For this review, take the finished solid that the model builds, in its own axes (mm). Face numbers are marked on the shaded views. A direction names the side the tool comes from. Round coordinates to 2 decimals unless told otherwise and drop trailing zeros. Write each loop counter-clockwise with the first axis right and the second up, starting at its lowest first coordinate (ties: lowest second). Pieces come first, ordered by that corner, then holes. Notation, with made-up numbers: (68, 47) -> (101, 47) arc R18 cw to (101, 63) -> close; hole circle Ø10 at (-11, 34). An arc over 180 degrees is marked (long way). Answer in a Markdown table with one row per item. Add a question column.
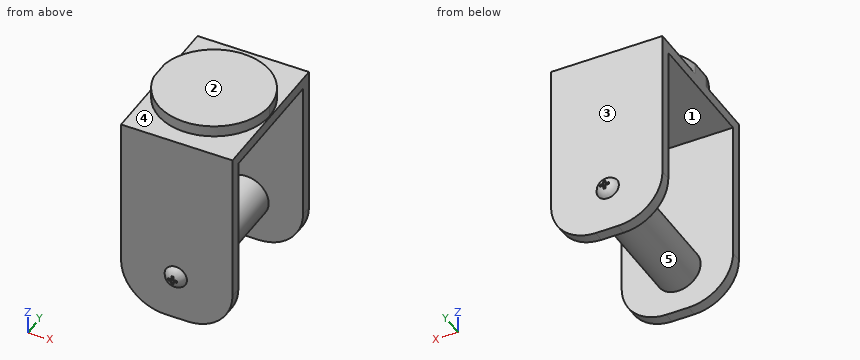
```python
from build123d import *

# Parameters (mm, degrees)
F1_DEPTH  = 5
F2_W      = 50
F2_H      = 55
F2_H_2    = 5
F3_DEPTH  = 5
F7_DEPTH  = 5
F8_R      = 10
F9_DEPTH  = 55
F10_R     = 5
F11_DEPTH = 3
F12_W     = 1.5
F12_H     = 1
F12_W_2   = 1
F12_H_2   = 1.5
F14_DEPTH = 3
F15_R     = 5
F16_DEPTH = 3
F18_DEPTH = 3


# Not quite as in the source:
# - a fillet or chamfer that OpenCascade refuses, or shapes differently, is made with other operations: its cross-section is extruded or revolved along the edge and cut away or added


with BuildPart() as f1:
    # F0 (on Front) → F1 (new body)
    with BuildSketch(Plane.XZ):
        with BuildLine():
            Line((25.4373252392, 36.0385786295), (-24.5626747608, 36.0385786295))
            Line((-24.5626747608, 36.0385786295), (-24.5626747608, -26.9614213705))
            ThreePointArc((-24.5626747608, -26.9614213705), (-18.7048103845, -41.1035569942), (-4.5626747608, -46.9614213705))
            Line((-4.5626747608, -46.9614213705), (5.4373252392, -46.9614213705))
            ThreePointArc((5.4373252392, -46.9614213705), (19.5794608629, -41.1035569942), (25.4373252392, -26.9614213705))
            Line((25.4373252392, -26.9614213705), (25.4373252392, 36.0385786295))
        make_face()
    extrude(amount=F1_DEPTH)

    # F2 (on face) → F3 (join)
    with BuildSketch(Plane.XY.offset(36.0385786295)):
        with Locations((0.4373252392, 27.5)):
            Rectangle(F2_W, F2_H)
        with Locations((0.4373252392, -2.5)):
            Rectangle(F2_W, F2_H_2)
    extrude(amount=F3_DEPTH)

    # F5: F1 across plane


with BuildPart() as f1_1:
    add(f1.part)
    add(f1.part.mirror(Plane(origin=(0.4373252392, 27.5, -3.8633044256), x_dir=(1, 0, 0), z_dir=(0, 1, 0))))

    # F6 (on face) → F7 (join)
    with BuildSketch(Plane.XY.offset(41.0385786295)):
        with BuildLine():
            ThreePointArc((-24.5626747608, 22.8443573382), (2.3380687521, 2.6095714278), (25, 27.5))
            ThreePointArc((25, 27.5), (2.3380687521, 52.3904285722), (-24.5626747608, 32.1556426618))
            Line((-24.5626747608, 32.1556426618), (-24.5626747608, 22.8443573382))
        make_face()
    extrude(amount=F7_DEPTH)

    # F8 (on face) → F9 (join, through all)
    with BuildSketch(Plane(origin=(0, 0, 0), x_dir=(-1, 0, 0), z_dir=(0, 1, 0))):
        with Locations((0, -26.9662032763)):
            Circle(F8_R)
    extrude(amount=F9_DEPTH)

    # F10 (on face) → F11 (join)
    with BuildSketch(Plane.XZ.offset(5)):
        with Locations((0, -26.4660866176)):
            Circle(F10_R)
    extrude(amount=F11_DEPTH)

    # F13: fillet of radius 5 on 1 edges, made by hand

    # F13_s1 → F13_t2 (revolve, cut)
    with BuildSketch(Plane.XY.offset(-26.4660866176)):
        with BuildLine():
            ThreePointArc((5, -5), (3.1560370926, -7.1833001327), (0.417424305, -8))
            Line((0.417424305, -8), (5, -8))
            Line((5, -8), (5, -5))
        make_face()
    revolve(axis=Axis((0, -8, -26.4660866176), (0, -1, 0)), mode=Mode.SUBTRACT)

    # F12 (on face) → F14 (cut)
    with BuildSketch(Plane.XZ.offset(8)):
        with Locations((-1.25, -26.4660866176)):
            Rectangle(F12_W, F12_H)
        Polygon((1, -25.9660866176), (0.5, -25.9660866176), (0.5, -26.9660866176), (1, -26.9660866176), (2, -26.9660866176), (2, -25.9660866176), align=None)
        with Locations((0, -26.4660866176)):
            Rectangle(F12_W_2, F12_H)
        with Locations((0, -25.2160866176)):
            Rectangle(F12_W_2, F12_H_2)
        with Locations((0, -27.7160866176)):
            Rectangle(F12_W_2, F12_H_2)
    extrude(amount=-F14_DEPTH, mode=Mode.SUBTRACT)

    # F15 (on face) → F16 (join)
    with BuildSketch(Plane(origin=(0, 60, 0), x_dir=(-1, 0, 0), z_dir=(0, 1, 0))):
        with Locations((0, -26.4660866176)):
            Circle(F15_R)
    extrude(amount=F16_DEPTH)

    # F17 (on face) → F18 (cut)
    with BuildSketch(Plane(origin=(0, 63, 0), x_dir=(-1, 0, 0), z_dir=(0, 1, 0))):
        Polygon((0.5, -24.4660866176), (-0.5, -24.4660866176), (-0.5, -25.9660866176), (-2, -25.9660866176), (-2, -26.9660866176), (-0.5, -26.9660866176), (-0.5, -28.4660866176), (0.5, -28.4660866176), (0.5, -26.9660866176), (2, -26.9660866176), (2, -25.9660866176), (0.5, -25.9660866176), align=None)
    extrude(amount=-F18_DEPTH, mode=Mode.SUBTRACT)

    # F19: fillet of radius 5 on 1 edges, made by hand

    # F19_s1 → F19_t2 (revolve, cut)
    with BuildSketch(Plane.XY.offset(-26.4660866176)):
        with BuildLine():
            ThreePointArc((-5, 60), (-3.1560370926, 62.1833001327), (-0.417424305, 63))
            Line((-0.417424305, 63), (-5, 63))
            Line((-5, 63), (-5, 60))
        make_face()
    revolve(axis=Axis((0, 63, -26.4660866176), (0, 1, 0)), mode=Mode.SUBTRACT)


solid = f1_1.part
```
1. We need section D-D (y = 29.5). Write out the cut boundary in (x, z), plus the area to 3 significant figures.
2. For L1, parallel to Y at x = -6, z = -9; L2, parallel to Z at x = -0.5, y = 45.5; L3, parallel to Z at x = 23.5, y = 29, list the stretches that pass through material, from the lowest coordinate up. Write a range as [from, to].
3. The part is to be moulded in two halves that separate along Y. For the marked faces 1, 2 and 3, say which applies: pulls with the +Y half, pulls with the -Y half, needs draft (parallel to the pull), parting line crosses it, or undercut.
4. Clearance check with flat-ended pins moving along their axes: pin 1 Ø0.8 at (x, y) = (0, 62) entering from +Z; pin 2 Ø10 at (x, z) = (-13.5, 30.5) entering from -Y; pin 3 Ø6 at (x, z) = (7.5, -7) entering from +Y. State where each tip first meets the part, or that it passes through.
5. Tool access review of the marked faces 4 and 5: name each direction out of +Z, -Z, +X, -X, +Y, -Y from which nothing blocks a thin tool from reaching the whole face with its end or side.
6. We need section A-A (y = 50). Write out the cut boundary in (x, z).
7. We need section C-C (z = -35). Write out the cut boundary in (x, y).
8. We need section B-B (x = -8.5). Write out the cut boundary in (y, z), plus the area to 3 significant figures.
Response:
| question | item | result |
|---|---|---|
| 1 | outline | (-24.56, 36.04) -> (25.44, 36.04) -> (25.44, 41.04) -> (24.92, 41.04) -> (24.92, 46.04) -> (-24.56, 46.04) -> close; circle Ø20 at (0, -26.97) |
| 1 | area | 812 mm2 |
| 2 | L1 | [-5, 0], [55, 60] |
| 2 | L2 | [-36.95, -16.98], [36.04, 46.04] |
| 2 | L3 | [36.04, 46.04] |
| 3 | face 1 | undercut |
| 3 | face 2 | needs draft |
| 3 | face 3 | pulls with the +Y half |
| 4 | pin 1 | z = -22.58 |
| 4 | pin 2 | y = -5 |
| 4 | pin 3 | y = 60 |
| 5 | face 4 | +Z |
| 5 | face 5 | none |
| 6 | outline | (-24.56, 36.04) -> (25.44, 36.04) -> (25.44, 41.04) -> (10.9, 41.04) -> (10.9, 46.04) -> (-10.9, 46.04) -> (-10.9, 41.04) -> (-24.56, 41.04) -> close; circle Ø20 at (0, -26.97) |
| 7 | outline | (-22.88, -5) -> (23.75, -5) -> (23.75, 0) -> (5.95, 0) -> (5.95, 55) -> (23.75, 55) -> (23.75, 60) -> (-22.88, 60) -> (-22.88, 55) -> (-5.95, 55) -> (-5.95, 0) -> (-22.88, 0) -> close |
| 8 | outline | (-5, -46.57) -> (0, -46.57) -> (0, -32.23) -> (55, -32.23) -> (55, -46.57) -> (60, -46.57) -> (60, 41.04) -> (51.01, 41.04) -> (51.01, 46.04) -> (3.99, 46.04) -> (3.99, 41.04) -> (-5, 41.04) -> close; hole (0, -21.7) -> (55, -21.7) -> (55, 36.04) -> (0, 36.04) -> close |
| 8 | area | 1,970 mm2 |
